Model file for the job. Use its own axes, mm. Coordinates: 2 decimals unless noted, no trailing zeros. Order: outer loops, then holes, each group sorted by start corner. A loop starts at its lowest first (then second) coordinate and runs counter-clockwise, first axis right, second up. Notation, with made-up numbers: (75.5, -13.5) -> (134.5, -13.5) arc R24 ccw to (134.5, 5.5) -> close; hole circle Ø11 at (84, 7). An arc over 180 degrees is marked (long way). Write item = value, one per line. Start each with the question number.
Q1. Wall check: line 1 (X direction, y = 13.75, z = 2.75); line 2 (Y direction, x = 10, z = 2.25); line 3 (X direction, y = 12.25, z = -4). Give the ranges that are in metal, low to high. Write a range as from..to.
Q2. Cut at C-C, the plane z = -6.5. List the corners of the cut face in (x, y), plus the area to 3 significant figures.
Q3. Cut at A-A, the plane y = 14. List the corners of the cut face in (x, z).
Q4. Cut at B-B, the plane x = 10. List the corners of the cut face in (y, z), plus the area to 3 significant figures.
Q5. Flat gauge pin, fed straight in: pin 1 (1.5 mm diameter, centred on x = 31.5, z = -5, fed in from -Y). Where does the tip first touch, or does it go through?
from build123d import *

# Parameters (mm, degrees)
SKETCH1_W             = 80
SKETCH1_H             = 19
BOSS_EXTRUDE1_DEPTH   = 10.5
M5X0_8_TAPPED_HOLE1_D = 4.2


with BuildPart() as part:
    # Sketch1 → Boss-Extrude1 (new, symmetric)
    with BuildSketch(Plane.XY):
        with Locations((40, 9.5)):
            Rectangle(SKETCH1_W, SKETCH1_H)
    extrude(amount=BOSS_EXTRUDE1_DEPTH, both=True)

    # M5x0.8 Tapped Hole1 (through all)
    with Locations(Plane.XY.offset(10.5)):
        with Locations((10, 14), (70, 14)):
            Hole(M5X0_8_TAPPED_HOLE1_D / 2)


solid = part.part
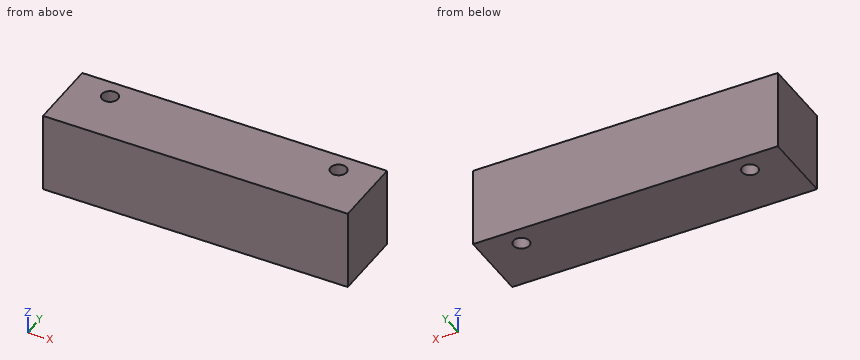
Here are the results:
q1.line_1 = 0..7.91, 12.09..67.91, 72.09..80
q1.line_2 = 0..11.9, 16.1..19
q1.line_3 = 0..8.84, 11.16..68.84, 71.16..80
q2.outline = (0, 0) -> (80, 0) -> (80, 19) -> (0, 19) -> close; hole circle Ø4.2 at (10, 14); hole circle Ø4.2 at (70, 14)
q2.area = 1,490 mm²
q3.outline = (0, -10.5) -> (7.9, -10.5) -> (7.9, 10.5) -> (0, 10.5) -> close; (12.1, -10.5) -> (67.9, -10.5) -> (67.9, 10.5) -> (12.1, 10.5) -> close; (72.1, -10.5) -> (80, -10.5) -> (80, 10.5) -> (72.1, 10.5) -> close
q4.outline = (0, -10.5) -> (11.9, -10.5) -> (11.9, 10.5) -> (0, 10.5) -> close; (16.1, -10.5) -> (19, -10.5) -> (19, 10.5) -> (16.1, 10.5) -> close
q4.area = 311 mm²
q5.pin_1 = 0
